Work out the finished part from the listing and answer in its coordinate system (mm). A direction names the side the tool comes from. Give positions to 0.01 mm unless a question says otherwise; leave off trailing zeros. Write each loop counter-clockwise with the first axis right and the second up, starting at its lowest first coordinate (ties: lowest second). Pieces come first, ordered by that corner, then holes. Notation, with made-up numbers: (49, 82.5) - (63, 82.5) arc R33 cw to (63, 116.5) - close; hole circle Ø1 at (15, 70). An arc over 180 degrees is marked (long way). Write item = value, one per line.
from build123d import *

# Parameters (mm, degrees)
SKETCH_1_R          = 5
EXTRUDE_1_DEPTH     = 10
CUT_EXTRUDE_1_DEPTH = 4
SKETCH_4_R          = 15
SKETCH_4_R_2        = 6
EXTRUDE_2_DEPTH     = 10
EXTRUDE_7_REACH     = 107.748
SKETCH_6_R          = 25
SKETCH_13_R         = 15
CUT_EXTRUDE_2_DEPTH = 109.800134443
FILLET_7_R          = 2
FILLET_8_R          = 2
FILLET_9_R          = 2
FILLET_10_R         = 1


with BuildPart() as part:
    # 草图1 → 凸台-拉伸1 (new body)
    with BuildSketch(Plane(origin=(0, 0, 0), x_dir=(1, 0, 0), z_dir=(0, 1, 0))):
        with BuildLine():
            Line((-52.5, 37.5), (52.5, 37.5))
            ThreePointArc((52.5, 37.5), (59.571067812, 34.571067812), (62.5, 27.5))
            Line((62.5, 27.5), (62.5, -27.5))
            ThreePointArc((62.5, -27.5), (59.571067812, -34.571067812), (52.5, -37.5))
            Line((52.5, -37.5), (-52.5, -37.5))
            ThreePointArc((-52.5, -37.5), (-59.571067812, -34.571067812), (-62.5, -27.5))
            Line((-62.5, -27.5), (-62.5, 27.5))
            ThreePointArc((-62.5, 27.5), (-59.571067812, 34.571067812), (-52.5, 37.5))
        make_face()
        with Locations(Location((-52.5, -27.5, 0), (0, 0, 270))):
            Circle(SKETCH_1_R, mode=Mode.SUBTRACT)
        with Locations(Location((52.5, -27.5, 0), (0, 0, 270))):
            Circle(SKETCH_1_R, mode=Mode.SUBTRACT)
        with Locations(Location((52.5, 27.5, 0), (0, 0, 270))):
            Circle(SKETCH_1_R, mode=Mode.SUBTRACT)
        with Locations(Location((-52.5, 27.5, 0), (0, 0, 270))):
            Circle(SKETCH_1_R, mode=Mode.SUBTRACT)
    extrude(amount=EXTRUDE_1_DEPTH)

    # 草图5 → 切除-拉伸1 (cut)
    with BuildSketch(Plane.XZ):
        with BuildLine():
            Line((40.5, 27.5), (-40.5, 27.5))
            ThreePointArc((-40.5, 27.5), (-44.014718626, 19.014718626), (-52.5, 15.5))
            Line((-52.5, 15.5), (-52.5, -15.5))
            ThreePointArc((-52.5, -15.5), (-44.014718626, -19.014718626), (-40.5, -27.5))
            Line((-40.5, -27.5), (40.5, -27.5))
            ThreePointArc((40.5, -27.5), (44.014718626, -19.014718626), (52.5, -15.5))
            Line((52.5, -15.5), (52.5, 15.5))
            ThreePointArc((52.5, 15.5), (44.014718626, 19.014718626), (40.5, 27.5))
        make_face()
    extrude(amount=-CUT_EXTRUDE_1_DEPTH, mode=Mode.SUBTRACT)

    # 草图4 → 凸台-拉伸2 (add)
    with BuildSketch(Plane(origin=(-19.955127019, 34.563293868, 0), x_dir=(0, 0, 1), z_dir=(-0.500000000000001, 0.866025403784438, 0))):
        with BuildLine():
            Line((30.98386677, 35.873412263), (52, 35.873412263))
            ThreePointArc((52, 35.873412263), (62, 25.873412263), (52, 15.873412263))
            Line((52, 15.873412263), (30.98386677, 15.873412263))
            ThreePointArc((30.98386677, 15.873412263), (28.814562191, 15.234084465), (27.338705973, 13.520471087))
            ThreePointArc((27.338705973, 13.520471087), (22.923803215, 6.52142926), (16.764705882, 0.994814299))
            ThreePointArc((16.764705882, 0.994814299), (15.468627995, -0.443659223), (15, -2.322332096))
            Line((15, -2.322332096), (15, -49.126587737))
            Line((15, -49.126587737), (-15, -49.126587737))
            Line((-15, -49.126587737), (-15, -2.322332096))
            ThreePointArc((-15, -2.322332096), (-15.468627995, -0.443659223), (-16.764705882, 0.994814299))
            ThreePointArc((-16.764705882, 0.994814299), (-19.351983004, 48.797215478), (27.338705973, 38.22635344))
            ThreePointArc((27.338705973, 38.22635344), (28.814562191, 36.512740062), (30.98386677, 35.873412263))
        make_face()
        with Locations(Location((0, 25.873412263, 0), (0, 0, 270))):
            Circle(SKETCH_4_R, mode=Mode.SUBTRACT)
        with Locations(Location((52, 25.873412263, 0), (0, 0, 270))):
            Circle(SKETCH_4_R_2, mode=Mode.SUBTRACT)
    extrude(amount=-EXTRUDE_2_DEPTH)

    # 凸台-拉伸7: up to this plane
    extrude_7_end = Plane(origin=(-52.5, 10, 27.5), z_dir=(0, 1, 0))
    # 草图6 → 凸台-拉伸7 (add, up to the surface)
    with BuildSketch(Plane(origin=(-14.955127019, 25.90303983, 0), x_dir=(0.8660254037844382, 0.500000000000001, 0), z_dir=(0.500000000000001, -0.8660254037844382, 0)), mode=Mode.PRIVATE) as extrude_7_sk1:
        with Locations(Location((25.873412263, 0, 0), (0, 0, 180))):
            Circle(SKETCH_6_R)
    extrude_7_tool1 = split(extrude(extrude_7_sk1.sketch, amount=EXTRUDE_7_REACH, mode=Mode.PRIVATE), bisect_by=extrude_7_end, keep=Keep.BOTH, mode=Mode.PRIVATE)
    add(extrude_7_tool1.solids().sort_by_distance((7.451905, 38.839746, 0))[0])

    # 草图13 → 切除-拉伸2 (cut, through all)
    with BuildSketch(Plane(origin=(-19.955127019, 34.563293868, 0), x_dir=(0, 0, 1), z_dir=(-0.500000000000001, 0.866025403784438, 0))):
        with Locations(Location((0, 25.873412263, 0), (0, 0, 270))):
            Circle(SKETCH_13_R)
    extrude(amount=-CUT_EXTRUDE_2_DEPTH, mode=Mode.SUBTRACT)

    # 圆角7
    fillet_7_edges = [part.edges().sort_by_distance(p)[0] for p in [
        (-52.5, 10, 15),
    ]]
    fillet(fillet_7_edges, radius=FILLET_7_R)

    # 圆角8
    # the kernel refuses this fillet: 2 mm, written as the material it adds along each edge
    with BuildSketch(Plane(origin=(-37.5, 10, -15), x_dir=(0, 0, -1), z_dir=(-1, 0, 0))) as fillet_8_piece_1_section:
        with BuildLine():
            CenterArc((FILLET_8_R, -FILLET_8_R), FILLET_8_R, 90, 90)
            Line((0, -FILLET_8_R), (0, 0))
            Line((0, 0), (FILLET_8_R, 0))
        make_face()
    fillet_8_piece_1 = extrude(amount=25, mode=Mode.PRIVATE)
    fillet_8_piece_1 = split(fillet_8_piece_1, bisect_by=Plane(origin=(-49.214592268, 6.123328347, -15.452717167), z_dir=(-0.500000000000001, 0.866025403784438, 0)), keep=Keep.TOP, mode=Mode.PRIVATE)
    fillet_8_piece_1 = split(fillet_8_piece_1, bisect_by=Plane(origin=(-54.214592268, 14.783582385, -15.452717167), z_dir=(0.500000000000001, -0.866025403784438, 0)), keep=Keep.TOP, mode=Mode.PRIVATE)
    add(fillet_8_piece_1)

    # 圆角9
    fillet_9_edges = [part.edges().sort_by_distance(p)[0] for p in [
        (52.970053814, 10, -0.001007854),
    ]]
    fillet(fillet_9_edges, radius=FILLET_9_R)

    # 圆角10
    fillet_10_edges = [part.edges().sort_by_distance(p)[0] for p in [
        (29.102540378, 51.339745962, 0),
    ]]
    fillet(fillet_10_edges, radius=FILLET_10_R)


solid = part.part
1. Find section A-A, the plane x = -50. Give the vertices of the cut face in (y, z).
Solution:
outline = (0, -37.5) - (10, -37.5) - (10, -31.83) - (0, -31.83) - close; (0, -23.17) - (10, -23.17) - (10, -17) arc R2 cw to (12, -15) - (17.22, -15) - (17.22, 15) - (12, 15) arc R2 cw to (10, 17) - (10, 23.17) - (0, 23.17) - (0, 15.76) - (4, 15.76) - (4, -15.76) - (0, -15.76) - close; (0, 31.83) - (10, 31.83) - (10, 37.5) - (0, 37.5) - close
2. Given pin 1 (5 mm diameter, centred on x = 15, y = 16.5, fed in from +Z); pin 2 (6.5 mm diameter, centred on x = -33.5, y = 20.5, fed in from +Z); pin 3 (1.2 mm diameter, centred on x = -16, y = 1.5, fed in from +Z), each flat-ended and moving along its own axis, determine where each tip first touches the part or whether it passes through.
Solution:
pin_1 = 24.91
pin_2 = 15
pin_3 = 37.5
3. Find section C-C, the plane z = 8. Give the number of separate pieces and of enclosed holes in the cut face, then the cut area to 3 significant figures.
Solution:
separate_pieces = 2
enclosed_holes = 1
area = 2,090 mm^2
4. A tool of negligible diameter and unlimited length cuts with its end or side. For faces 1 (the flat face through (13.577, 48.23, 41.345)), 2 (the flat face through (-3.743, 38.23, 41.639)), 3 (the flat face through (-52.5, 2, 0)), from which of +Z, -Z, +X, -X, +Y, -Y can it reach the whole face along a straight path? Write none if from no direction.
Solution:
face_1 = +Z, +X, +Y
face_2 = +Z, -X
face_3 = -Y
5. For a pull along X with two mould halves and no side action, classify faces 4 (the cylindrical face through (26.74, 35.4, 0.66)), 5 (the flat face through (-34, 21, -15)), 6 (the flat face through (-13, 10, -1)), 7 (the flat face through (-62.5, 5, 0)) as pulls with the +X half, pulls with the -X half, needs draft (parallel to the pull), parting line crosses it, or undercut.
Solution:
face_4 = undercut
face_5 = needs draft
face_6 = undercut
face_7 = pulls with the -X half
6. Find section B-B, the plane z = 49.5. Give the vertices of the cut face in (x, y).
Solution:
outline = (-6.21, 42.5) - (-1.21, 33.84) - (2.73, 36.11) - (-2.27, 44.77) - close; (7.18, 50.23) - (12.18, 41.57) - (16.11, 43.84) - (11.11, 52.5) - close
7. Straight lines are drawn through the part: line 1 (X direction, y = 5.75, z = -27.5); line 2 (Z direction, x = 52, y = 8); line 3 (Z direction, x = -41.5, y = 18.5). For each, find the intervals that lie inside material, in ascending order.
Solution:
line_1 = -62.5 to -57.5, -47.5 to 47.5, 57.5 to 62.5
line_2 = -37.5 to -32.47, -22.53 to 22.53, 32.47 to 37.5
line_3 = -15 to 15
